```python
from build123d import *

# Parameters (mm, degrees)
BOSS_EXTRU_1_DEPTH        = 33.175
BOSS_EXTRU_1_DEPTH_BACK   = 3.175
BOSS_EXTRU_1_2_DEPTH      = 33.175
BOSS_EXTRU_1_2_DEPTH_BACK = 3.175
BOSS_EXTRU_1_3_DEPTH      = 33.175
BOSS_EXTRU_1_3_DEPTH_BACK = 3.175
BOSS_EXTRU_1_4_DEPTH      = 33.175
BOSS_EXTRU_1_4_DEPTH_BACK = 3.175
BOSS_EXTRU_1_5_DEPTH      = 33.175
BOSS_EXTRU_1_5_DEPTH_BACK = 3.175
BOSS_EXTRU_1_6_DEPTH      = 33.175
BOSS_EXTRU_1_6_DEPTH_BACK = 3.175
BOSS_EXTRU_1_7_DEPTH      = 33.175
BOSS_EXTRU_1_7_DEPTH_BACK = 3.175
BOSS_EXTRU_2_DEPTH        = 198.346
BOSS_EXTRU_2_DEPTH_BACK   = 218.854
ESQUISSE2_W               = 3.175
ESQUISSE2_H               = 30
CUT_EXTRUDE1_REACH        = 213.245
SKETCH1_R                 = 8.75
LPATTERN1_COUNT           = 14
LPATTERN1_PITCH           = 29.785


with BuildPart() as part:
    # Esquisse1 → Boss.-Extru.1 (new, two sides: drawn at the far end of the back side and taken through both)
    with BuildSketch(Plane.XY.offset(-BOSS_EXTRU_1_DEPTH_BACK)):
        Polygon((-56, 163.6), (-56, 163.346), (-52.825, 163.346), (-52.825, 163.6), (-52.825, 183.6), (-52.825, 183.854), (-56, 183.854), (-56, 183.6), align=None)
    extrude(amount=BOSS_EXTRU_1_DEPTH + BOSS_EXTRU_1_DEPTH_BACK)



with BuildPart() as body_2:
    # Esquisse1 → Boss.-Extru.1 2 (new, two sides: drawn at the far end of the back side and taken through both)
    with BuildSketch(Plane.XY.offset(-BOSS_EXTRU_1_2_DEPTH_BACK)):
        Polygon((-56, 125.733333333), (-56, 125.987333333), (-52.825, 125.987333333), (-52.825, 125.733333333), (-52.825, 105.733333333), (-52.825, 105.479333333), (-56, 105.479333333), (-56, 105.733333333), align=None)
    extrude(amount=BOSS_EXTRU_1_2_DEPTH + BOSS_EXTRU_1_2_DEPTH_BACK)


with BuildPart() as body_3:
    # Esquisse1 → Boss.-Extru.1 3 (new, two sides: drawn at the far end of the back side and taken through both)
    with BuildSketch(Plane.XY.offset(-BOSS_EXTRU_1_3_DEPTH_BACK)):
        Polygon((-56, 67.866666667), (-56, 68.120666667), (-52.825, 68.120666667), (-52.825, 67.866666667), (-52.825, 47.866666667), (-52.825, 47.612666667), (-56, 47.612666667), (-56, 47.866666667), align=None)
    extrude(amount=BOSS_EXTRU_1_3_DEPTH + BOSS_EXTRU_1_3_DEPTH_BACK)


with BuildPart() as body_4:
    # Esquisse1 → Boss.-Extru.1 4 (new, two sides: drawn at the far end of the back side and taken through both)
    with BuildSketch(Plane.XY.offset(-BOSS_EXTRU_1_4_DEPTH_BACK)):
        Polygon((-56, 10), (-56, 10.254), (-52.825, 10.254), (-52.825, 10), (-52.825, -10), (-52.825, -10.254), (-56, -10.254), (-56, -10), align=None)
    extrude(amount=BOSS_EXTRU_1_4_DEPTH + BOSS_EXTRU_1_4_DEPTH_BACK)


with BuildPart() as body_5:
    # Esquisse1 → Boss.-Extru.1 5 (new, two sides: drawn at the far end of the back side and taken through both)
    with BuildSketch(Plane.XY.offset(-BOSS_EXTRU_1_5_DEPTH_BACK)):
        Polygon((-56, -163.6), (-56, -183.6), (-56, -183.854), (-52.825, -183.854), (-52.825, -183.6), (-52.825, -163.6), (-52.825, -163.346), (-56, -163.346), align=None)
    extrude(amount=BOSS_EXTRU_1_5_DEPTH + BOSS_EXTRU_1_5_DEPTH_BACK)


with BuildPart() as body_6:
    # Esquisse1 → Boss.-Extru.1 6 (new, two sides: drawn at the far end of the back side and taken through both)
    with BuildSketch(Plane.XY.offset(-BOSS_EXTRU_1_6_DEPTH_BACK)):
        Polygon((-56, -105.733333333), (-56, -125.733333333), (-56, -125.987333333), (-52.825, -125.987333333), (-52.825, -125.733333333), (-52.825, -105.733333333), (-52.825, -105.479333333), (-56, -105.479333333), align=None)
    extrude(amount=BOSS_EXTRU_1_6_DEPTH + BOSS_EXTRU_1_6_DEPTH_BACK)


with BuildPart() as body_7:
    # Esquisse1 → Boss.-Extru.1 7 (new, two sides: drawn at the far end of the back side and taken through both)
    with BuildSketch(Plane.XY.offset(-BOSS_EXTRU_1_7_DEPTH_BACK)):
        Polygon((-56, -47.866666667), (-56, -67.866666667), (-56, -68.120666667), (-52.825, -68.120666667), (-52.825, -67.866666667), (-52.825, -47.866666667), (-52.825, -47.612666667), (-56, -47.612666667), align=None)
    extrude(amount=BOSS_EXTRU_1_7_DEPTH + BOSS_EXTRU_1_7_DEPTH_BACK)


with BuildPart() as part_1:
    add(part.part)

    add(body_2.part)  # Boss.-Extru.2 merges body 2

    add(body_3.part)  # Boss.-Extru.2 merges body 3

    add(body_4.part)  # Boss.-Extru.2 merges body 4

    add(body_5.part)  # Boss.-Extru.2 merges body 5

    add(body_6.part)  # Boss.-Extru.2 merges body 6

    add(body_7.part)  # Boss.-Extru.2 merges body 7
    # Esquisse2 → Boss.-Extru.2 (add, two sides: drawn at the far end of the back side and taken through both)
    with BuildSketch(Plane.XZ.offset(10.254).offset(-BOSS_EXTRU_2_DEPTH_BACK)):
        with Locations((-54.4125, 15)):
            Rectangle(ESQUISSE2_W, ESQUISSE2_H)
    extrude(amount=BOSS_EXTRU_2_DEPTH + BOSS_EXTRU_2_DEPTH_BACK)

    # Sketch1 → Cut-Extrude1 (cut, up to next)
    with BuildSketch(Plane(origin=(-52.825000001, 0, 0), x_dir=(0, 0, -1), z_dir=(1.0, 8.38677334054915e-12, 0)), mode=Mode.PRIVATE) as cut_extrude1_sk1:
        with Locations(Location((-15, -193.6, 0), (0, 0, 90))):
            Circle(SKETCH1_R)
    cut_extrude1_tool1 = extrude(cut_extrude1_sk1.sketch, amount=-CUT_EXTRUDE1_REACH, mode=Mode.PRIVATE) & part_1.part
    cut_extrude1 = cut_extrude1_tool1.solids().sort_by_distance((-52.825, -193.6, 15))[0]
    add(cut_extrude1, mode=Mode.SUBTRACT)

    # LPattern1: Cut-Extrude1 ×14
    with Locations(*[(0, i * LPATTERN1_PITCH, 0) for i in range(1, LPATTERN1_COUNT)]):
        add(cut_extrude1, mode=Mode.SUBTRACT)


solid = part_1.part
```
CAD build for the part. Positions are in the model's coordinates, mm. Coordinates: 2 decimals unless noted, no trailing zeros. Order: outer loops, then holes, each group sorted by start corner. A loop starts at its lowest first (then second) coordinate and runs counter-clockwise, first axis right, second up. Notation, with made-up numbers: (53, 63.25) - (103, 63.25) arc R21 cw to (103, 75.25) - close; hole circle Ø4 at (49.25, -8). An arc over 180 degrees is marked (long way). Use a Markdown table: item, result. Add a question column.
(1) Pull direction Y, two halves, no side cores. Call faces 1 (the face through (-52.825, 3, 15)), 2 (the face through (-54.39, 53.026, 17.628)): +Y half, -Y half, draft (parallel to the pull), parting line (faces both ways), or undercut.
(2) Drill centre lines: line 1 along Z through (x, y) = (-54.55, -134.03); line 2 along Z through (x, y) = (-54.1, 163.82) (3 decimals). Where is each one in solid material? Low to high. Write a range as [from, to].
(3) Saw through at A-A (y = -74.46). Give the cut face in (x, z) (3 decimals), then the cut area to 3 significant figures.
(4) Saw through at B-B (x = -53.4). Count the separate pieces of the cut face and the enclosed holes in it, then the cut area to 3 significant figures.
(5) Flat gauge pins, fed straight in: pin 1 (1 mm diameter, centred on x = -54, z = 32, fed in from +Y); pin 2 (1.6 mm diameter, centred on x = -55, y = -201.5, fed in from -Z); pin 3 (1.6 mm diameter, centred on x = -55, z = 31, fed in from -Y). Where does each tip first touch, or does it go through?
Solved:
| question | item | result |
|---|---|---|
| 1 | face 1 | draft |
| 1 | face 2 | undercut |
| 2 | line 1 | z = [0, 6.25], [23.75, 30] |
| 2 | line 2 | z = [-3.175, 6.25], [23.75, 33.175] |
| 3 | outline | (-56, 0) - (-52.825, 0) - (-52.825, 6.25) - (-56, 6.25) - close; (-56, 23.75) - (-52.825, 23.75) - (-52.825, 30) - (-56, 30) - close |
| 3 | area | 39.7 mm² |
| 4 | separate pieces | 1 |
| 4 | enclosed holes | 14 |
| 4 | area | 10,100 mm² |
| 5 | pin 1 | stops at y = 183.85 |
| 5 | pin 2 | stops at z = 0 |
| 5 | pin 3 | stops at y = -183.85 |
